Could you check a few things on this model? Use its own coordinates, in mm. Coordinates: 2 decimals unless noted, no trailing zeros. Order: outer loops, then holes, each group sorted by start corner. A loop starts at its lowest first (then second) coordinate and runs counter-clockwise, first axis right, second up. Notation, with made-up numbers: (-22.75, 4.25) -> (-16.75, 4.25) arc R5 ccw to (-16.75, 10.25) -> close; hole circle Ø6 at (-18.75, -19). An arc over 180 degrees is marked (long way). Use a Markdown table: item, result. Add a question column.
1) Will these pins go through, and if not, where does the flat tip stop? pin 1 Ø1 at (y, z) = (-3, 215) entering from +X; pin 2 Ø0.6 at (x, z) = (103, 214.5) entering from -Y; pin 3 Ø1.6 at (x, y) = (86.5, -5) entering from -Z.
2) If we section it at A-A (x = 191.5): Write out the boundary of the cut face in (y, z), plus the area to 3 significant figures.
3) If I drill on L1, parallel to Z at x = 84, y = -8.5; L2, parallel to Y at x = 207.5, z = 215; L3, parallel to X at y = -3.5, z = 214, over which ranges is the centre line in solid material (lowest first)? Write a range as [from, to].
```python
from build123d import *

# Parameters (mm, degrees)
CROQUIS2_W                   = 220
CROQUIS2_H                   = 220
CROQUIS2_W_2                 = 200
CROQUIS2_H_2                 = 200
SALIENTE_EXTRUIR1_DEPTH      = 10
CROQUIS3_W                   = 212
CROQUIS3_H                   = 212
CROQUIS3_W_2                 = 210
CROQUIS3_H_2                 = 210
CROQUIS3_W_3                 = 208
CROQUIS3_H_3                 = 208
CORTAR_EXTRUIR1_DEPTH        = 3.5
CROQUIS4_W                   = 10
CROQUIS4_H                   = 10
SALIENTE_EXTRUIR2_DEPTH      = 200
SALIENTE_EXTRUIR2_DEPTH_BACK = 10
CROQUIS6_W                   = 3.5
CROQUIS6_H                   = 2
CROQUIS6_W_2                 = 2
CROQUIS6_H_2                 = 3.5
CROQUIS6_W_3                 = 1.99805467
CORTAR_EXTRUIR2_DEPTH        = 203.5
CROQUIS7_W                   = 220
CROQUIS7_H                   = 220
CROQUIS7_W_2                 = 200
CROQUIS7_H_2                 = 200
SALIENTE_EXTRUIR3_DEPTH      = 10
CORTAR_EXTRUIR3_START        = -3.5
CROQUIS8_W                   = 207
CROQUIS8_H                   = 2
CORTAR_EXTRUIR3_DEPTH        = 207
MATRIZC1_COUNT               = 4
CROQUIS9_W                   = 86
CROQUIS9_H                   = 16
BRAZOS_DEPTH                 = 10
MATRIZC2_COUNT               = 4
CORTAR_EXTRUIR4_DEPTH        = 221
CORTAR_EXTRUIR6_DEPTH        = 11
CROQUIS12_R                  = 3.1
CORTAR_EXTRUIR7_DEPTH        = 10.2
CROQUIS13_R                  = 3.1
CORTAR_EXTRUIR8_DEPTH        = 10.2


with BuildPart() as part:
    # Croquis2 → Saliente-Extruir1 (new body)
    with BuildSketch(Plane.XY):
        with Locations((110, -110)):
            Rectangle(CROQUIS2_W, CROQUIS2_H)
        with Locations((110, -110)):
            Rectangle(CROQUIS2_W_2, CROQUIS2_H_2, mode=Mode.SUBTRACT)
    extrude(amount=SALIENTE_EXTRUIR1_DEPTH)

    # Croquis3 → Cortar-Extruir1 (cut)
    with BuildSketch(Plane.XY.offset(10)):
        with Locations((110, -110)):
            Rectangle(CROQUIS3_W, CROQUIS3_H)
        with Locations((110, -110)):
            Rectangle(CROQUIS3_W_2, CROQUIS3_H_2, mode=Mode.SUBTRACT)
        with Locations((110, -110)):
            Rectangle(CROQUIS3_W_2, CROQUIS3_H_2)
        with Locations((110, -110)):
            Rectangle(CROQUIS3_W_3, CROQUIS3_H_3, mode=Mode.SUBTRACT)
    extrude(amount=-CORTAR_EXTRUIR1_DEPTH, mode=Mode.SUBTRACT)

    # Croquis4 → Saliente-Extruir2 (add, two sides)
    with BuildSketch(Plane.XY.offset(10)) as saliente_extruir2_sk:
        with Locations((5, -5)):
            Rectangle(CROQUIS4_W, CROQUIS4_H)
        with Locations((215, -5)):
            Rectangle(CROQUIS4_W, CROQUIS4_H)
        with Locations((215, -215)):
            Rectangle(CROQUIS4_W, CROQUIS4_H)
        with Locations((5, -215)):
            Rectangle(CROQUIS4_W, CROQUIS4_H)
    extrude(amount=SALIENTE_EXTRUIR2_DEPTH)
    extrude(saliente_extruir2_sk.sketch, amount=-SALIENTE_EXTRUIR2_DEPTH_BACK)

    # Croquis6 → Cortar-Extruir2 (cut)
    with BuildSketch(Plane.XY.offset(210)):
        with Locations((8.25, -5)):
            Rectangle(CROQUIS6_W, CROQUIS6_H)
        with Locations((5, -8.25)):
            Rectangle(CROQUIS6_W_2, CROQUIS6_H_2)
        with Locations((211.75, -5)):
            Rectangle(CROQUIS6_W, CROQUIS6_H)
        with Locations((215, -8.25)):
            Rectangle(CROQUIS6_W_2, CROQUIS6_H_2)
        with Locations((211.75, -215)):
            Rectangle(CROQUIS6_W, CROQUIS6_H)
        with Locations((215.000972665, -211.75)):
            Rectangle(CROQUIS6_W_3, CROQUIS6_H_2)
        with Locations((5, -211.75)):
            Rectangle(CROQUIS6_W_2, CROQUIS6_H_2)
        with Locations((8.25, -215)):
            Rectangle(CROQUIS6_W, CROQUIS6_H)
    extrude(amount=-CORTAR_EXTRUIR2_DEPTH, mode=Mode.SUBTRACT)

    # Croquis7 → Saliente-Extruir3 (add)
    with BuildSketch(Plane.XY.offset(210)):
        with Locations((110, -110)):
            Rectangle(CROQUIS7_W, CROQUIS7_H)
        with Locations((110, -110)):
            Rectangle(CROQUIS7_W_2, CROQUIS7_H_2, mode=Mode.SUBTRACT)
    extrude(amount=SALIENTE_EXTRUIR3_DEPTH)

    # Croquis8 → Cortar-Extruir3 (cut)
    with BuildSketch(Plane(origin=(0, -210, 0), x_dir=(1, 0, 0), z_dir=(0, 1, 0)).offset(CORTAR_EXTRUIR3_START)):
        with Locations((110, -215)):
            Rectangle(CROQUIS8_W, CROQUIS8_H)
    cortar_extruir3 = extrude(amount=CORTAR_EXTRUIR3_DEPTH, mode=Mode.SUBTRACT)

    # MatrizC1: Cortar-Extruir3 ×4 about axis
    matrizc1_axis = Axis((0, -110, 110), (1, 0, 0))
    for i in range(1, MATRIZC1_COUNT):
        add(cortar_extruir3.rotate(matrizc1_axis, i * 360 / MATRIZC1_COUNT), mode=Mode.SUBTRACT)

    # Croquis9 → Brazos (add)
    with BuildSketch(Plane.XY.offset(220)):
        with Locations((43, -110)):
            Rectangle(CROQUIS9_W, CROQUIS9_H)
        with BuildLine():
            ThreePointArc((71.801526277, -112.25), (69.551526277, -110), (71.801526277, -107.75))
            Line((71.801526277, -107.75), (75, -107.75))
            ThreePointArc((75, -107.75), (77.25, -110), (75, -112.25))
            Line((75, -112.25), (71.801526277, -112.25))
        make_face(mode=Mode.SUBTRACT)
        with Locations((177, -110)):
            Rectangle(CROQUIS9_W, CROQUIS9_H)
        with BuildLine():
            Line((145, -107.75), (148.198473723, -107.75))
            ThreePointArc((148.198473723, -107.75), (150.448473723, -110), (148.198473723, -112.25))
            Line((148.198473723, -112.25), (145, -112.25))
            ThreePointArc((145, -112.25), (142.75, -110), (145, -107.75))
        make_face(mode=Mode.SUBTRACT)
    extrude(amount=-BRAZOS_DEPTH)

    # MatrizC2: Cortar-Extruir3 ×4 about axis
    matrizc2_axis = Axis((110, 0, 110), (0, 1, 0))
    for i in range(1, MATRIZC2_COUNT):
        add(cortar_extruir3.rotate(matrizc2_axis, i * 360 / MATRIZC2_COUNT), mode=Mode.SUBTRACT)

    # Croquis10 → Cortar-Extruir4 (cut, through all)
    with BuildSketch(Plane(origin=(0, 0, 0), x_dir=(1, 0, 0), z_dir=(0, 1, 0))):
        Polygon((210, -210), (-54.613887122, -210), (-54.613887122, 5.730335669), (210, 5.730335669), (296.699829043, 5.730335669), (296.699829043, -210), align=None)
    extrude(amount=-CORTAR_EXTRUIR4_DEPTH, mode=Mode.SUBTRACT)

    # Croquis11 → Cortar-Extruir6 (cut, through all)
    with BuildSketch(Plane.XY.offset(220)):
        Polygon((225.348159566, -10), (300.018724731, -10), (300.018724731, -229.853044827), (10, -229.853044827), (-53.650825238, -229.853044827), (-53.650825238, -10), (-6.520912183, -10), (-6.520912183, 9.079623398), (10, 9.079623398), (10, -10), (210, -10), (210, 9.87282219), (225.348159566, 9.87282219), align=None)
    extrude(amount=-CORTAR_EXTRUIR6_DEPTH, mode=Mode.SUBTRACT)

    # Croquis12 → Cortar-Extruir7 (cut)
    with BuildSketch(Plane.ZY.offset(-10)):
        with Locations((215, -5)):
            Circle(CROQUIS12_R)
    extrude(amount=-CORTAR_EXTRUIR7_DEPTH, mode=Mode.SUBTRACT)

    # Croquis13 → Cortar-Extruir8 (cut)
    with BuildSketch(Plane(origin=(210, 0, 0), x_dir=(0, 0, -1), z_dir=(1, 0, 0))):
        with Locations((-215, -5)):
            Circle(CROQUIS13_R)
    extrude(amount=-CORTAR_EXTRUIR8_DEPTH, mode=Mode.SUBTRACT)


solid = part.part
```
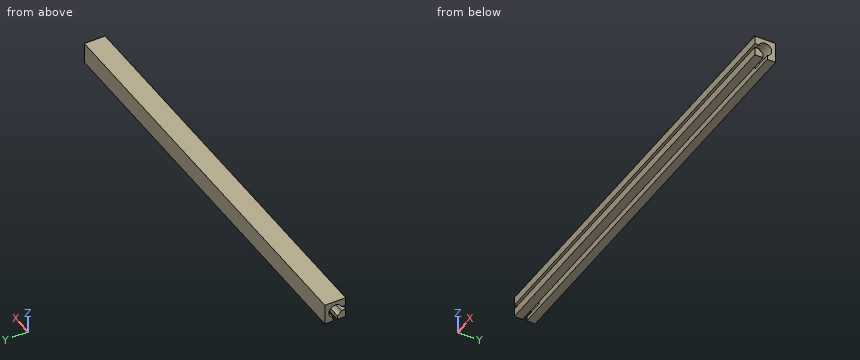
Answer sheet:
| question | item | result |
|---|---|---|
| 1 | pin 1 | x = 199.8 |
| 1 | pin 2 | y = -6.5 |
| 1 | pin 3 | z = 213.5 |
| 2 | outline | (-10, 210) -> (-6, 210) -> (-6, 213.5) -> (-4, 213.5) -> (-4, 210) -> (0, 210) -> (0, 220) -> (-10, 220) -> (-10, 216) -> (-6.5, 216) -> (-6.5, 214) -> (-10, 214) -> close |
| 2 | area | 86.0 mm2 |
| 3 | L1 | [210, 214], [216, 220] |
| 3 | L2 | [-1.9, 0] |
| 3 | L3 | [20.2, 199.8] |
